CAD build for the part. Positions are in the model's coordinates, mm. A direction names the side the tool comes from. Round coordinates to 2 decimals unless told otherwise and drop trailing zeros. Loops run counter-clockwise (first coordinate to the right, second up) from the corner with the lowest first, then second, coordinate; pieces in that order, holes last.
```python
from build123d import *

# Parameters (mm, degrees)
SKETCH1_R           = 4
BOSS_EXTRUDE1_DEPTH = 114.3
BOSS_EXTRUDE2_DEPTH = 35
CUT_EXTRUDE1_DEPTH  = 5.596433308


with BuildPart() as part:
    # Sketch1 → Boss-Extrude1 (new body)
    with BuildSketch(Plane.XY):
        Circle(SKETCH1_R)
    extrude(amount=BOSS_EXTRUDE1_DEPTH)

    # Sketch2 → Boss-Extrude2 (add)
    with BuildSketch(Plane.XY.offset(114.3)):
        Polygon((-1.2954, 3.421433318), (-1.2954, 6.421433318), (1.2954, 6.421433318), (1.2954, 3.421433318), (1.2954, 0.825), (0, 0.825), (-1.2954, 0.825), align=None)
    extrude(amount=-BOSS_EXTRUDE2_DEPTH)

    # Sketch3 → Cut-Extrude1 (cut)
    with BuildSketch(Plane(origin=(0, 6.421433318, 0), x_dir=(1, 0, 0), z_dir=(0, 1, 0))):
        with BuildLine():
            Line((-1.2954, -79.3), (-1.2954, -114.3))
            Line((-1.2954, -114.3), (1.2954, -114.3))
            Line((1.2954, -114.3), (1.2954, -79.3))
            ThreePointArc((1.2954, -79.3), (0, -78.0046), (-1.2954, -79.3))
        make_face()
    extrude(amount=-CUT_EXTRUDE1_DEPTH, mode=Mode.SUBTRACT)


solid = part.part
```
Item 1: Cut at C-C, the plane y = -1.5. Give the cut face in (x, z), plus the area to 3 significant figures.
Answers follow:
outline: (-3.71, 0) - (3.71, 0) - (3.71, 114.3) - (-3.71, 114.3) - close
area: 848 mm2
Item 2: Flat gauge pins, fed straight in: P1, Ø3, axis at x = 0, z = 104.5, coming from the +Y side; P2, Ø3.5, axis at y = 2.5, z = 89, coming from the -X side; P3, Ø1.5, axis at x = 1.5, z = 91.5, coming from the -Y side. Where does each tip first touch, or does it go through?
Answers follow:
P1: stops at y = 3.78
P2: stops at x = -3.93
P3: stops at y = -3.93
Item 3: Cut at B-B, the plane z = 50.5. Give the cut face in (x, y).
Answers follow:
outline: circle Ø8 at (0, 0)
Item 4: Probe line 1 (X direction, y = 2.5, z = 103.5); line 2 (X direction, y = -2.5, z = 66.5); line 3 (Y direction, x = -0.25, z = 76). List the from-to ranges inside material, lowest first.
Answers follow:
line 1: x = -3.12 to -1.3, 1.3 to 3.12
line 2: x = -3.12 to 3.12
line 3: y = -3.99 to 3.99
Item 5: Cut at A-A, the plane x = 0. Give the cut face in (y, z) (3 decimals), plus the area to 3 significant figures.
Answers follow:
outline: (-4, 0) - (4, 0) - (4, 78.005) - (0.825, 78.005) - (0.825, 114.3) - (-4, 114.3) - close
area: 799 mm2
Item 6: 3-axis set-ups, long thin cutter, end or side, ignore diameter. For faces 1 (the flat face through (0, 0, 114.3)), 2 (the cylindrical face through (0.028, 2.437, 78.005)): which of +Z, -Z, +X, -X, +Y, -Y reach the whole face in a straight line?
Answers follow:
face 1: +Z, +X, -X, +Y, -Y
face 2: +Z, +Y
Item 7: Cut at D-D, the plane z = 104. Give the cut face in (x, y) (3 decimals).
Answers follow:
outline: (-1.295, 0.825) - (-1.295, 3.784) arc R4 ccw (long way) to (1.295, 3.784) - (1.295, 0.825) - close
